Read the model definition and answer for the solid it produces. Units are mm, in the model's axes. Give positions to 0.01 mm unless a question says otherwise; leave off trailing zeros. Write each loop counter-clockwise with the first axis right and the second up, starting at its lowest first coordinate (ties: lowest second). Pieces come first, ordered by that corner, then holes. Notation, with made-up numbers: (76.5, 41.5) -> (132.5, 41.5) arc R23 ccw to (132.5, 77.5) -> close; hole circle Ø1 at (-3, 15.5). An arc over 180 degrees is marked (long way). Answer as CSV lines item,"result". Start each with the question number.
1. The part is cut by section C-C, the plane x = 191. Determine the outline of the cut face in (y, z).
2. Given pin 1 (8 mm diameter, centred on x = 167, y = -2, fed in from +Z); pin 2 (1 mm diameter, centred on x = 130.5, y = -12.5, fed in from +Z); pin 3 (8 mm diameter, centred on y = -3, z = 75, fed in from +X), each flat-ended and moving along its own axis, determine where each tip first touches the part or whether it passes through.
3. The part is cut by section A-A, the plane y = -8.25. Determine the outline of the cut face in (x, z), and give its area (4 significant figures).
4. Find the intervals of material crossed by line 1 (X direction, y = -2.75, z = -51); line 2 (X direction, y = -3.25, z = -8.5); line 3 (Z direction, x = 293.5, y = -10.75), in increasing order.
5. The part is cut by section B-B, the plane z = 66. Determine the outline of the cut face in (x, y).
from build123d import *

# Parameters (mm, degrees)
F1_DEPTH = 18


# Not quite as in the source:
# - a feature names something its author has since deleted; it is built from what else it names


with BuildPart() as f1:
    # F0 (on Front) → F1 (new body)
    with BuildSketch(Plane.XZ):
        Polygon((310, -100), (100, 200), (100, -100), align=None)
        Polygon((-100, 200), (-100, -200), (100, -200), (310, -200), (310, -100), (100, -100), (100, 200), align=None)
    extrude(amount=F1_DEPTH)


solid = f1.part
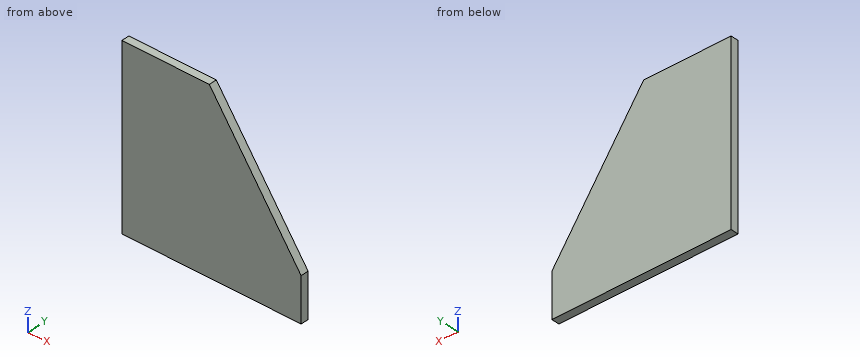
Results found:
1,outline,"(-18, -200) -> (0, -200) -> (0, 70) -> (-18, 70) -> close"
2,pin 1,"stops at z = 110"
2,pin 2,"stops at z = 157.14"
2,pin 3,"stops at x = 190.3"
3,outline,"(-100, -200) -> (310, -200) -> (310, -100) -> (100, 200) -> (-100, 200) -> close"
3,area,"132,500 mm²"
4,line 1,"x = -100 to 275.7"
4,line 2,"x = -100 to 245.95"
4,line 3,"z = -200 to -76.43"
5,outline,"(-100, -18) -> (193.8, -18) -> (193.8, 0) -> (-100, 0) -> close"
